Check sheet for the modelled part. Datum: model origin and axes. Units: mm. Face numbers are marked on the shaded views. A direction names the side the tool comes from. Round coordinates to 2 decimals unless told otherwise and drop trailing zeros. Loops run counter-clockwise (first coordinate to the right, second up) from the corner with the lowest first, then second, coordinate; pieces in that order, holes last. Notation, with made-up numbers: (45.25, 14) -> (99.25, 14) arc R7 ccw to (99.25, 26) -> close; hole circle Ø8 at (-3, -20). An arc over 180 degrees is marked (long way). Use one line per item in the form item = value. Start each with the question number.
(1) Material ranges on probe 1 along Y at (x, z) = (-8.5, 9.75); probe 2 along Z at (x, y) = (6, 20.5); probe 3 along Z at (x, y) = (8, 27.5), recorded low to high. Write a range as [from, to].
(2) Sectioned sample at B-B (y = 41). Record the cut outline in (x, z), and give its area (3 significant figures).
(3) Go/stop test with flat-tipped pins: pin 1 (10 mm diameter, centred on y = 20, z = 0.5, fed in from +X); pin 2 (12 mm diameter, centred on y = 39.5, z = -0.5, fed in from +X); pin 3 (2 mm diameter, centred on y = 35.5, z = -0.5, fed in from +X); pin 4 (14.5 mm diameter, centred on x = 8, z = 1, fed in from +Y). Record where each tip stops, or that it passes through.
(4) Set-up check for the marked faces 1, 2 and 3: record each of +Z, -Z, +X, -X, +Y, -Y from which the full face is reachable in a straight line by a thin tool's end or side.
(5) Sectioned sample at D-D (x = 10). Record the cut outline in (y, z).
(6) Draft check along Z on the marked faces 4, 5 and 6. Enter one of: released by +Z, released by -Z, zero draft, split by the parting line, or undercut.
(7) Sectioned sample at C-C (z = -2.25). Record the cut outline in (x, y).
(8) Sectioned sample at A-A (x = 3). Record the cut outline in (y, z).
from build123d import *

# Parameters (mm, degrees)
EXTRUDE_1_DEPTH = 3
EXTRUDE_START   = -3
EXTRUDE_2_DEPTH = 63
EXTRUDE_3_DEPTH = 3


with BuildPart() as part:
    # 草图1 → 凸台-拉伸1 (new body)
    with BuildSketch(Plane(origin=(0, 0, 0), x_dir=(1, 0, 0), z_dir=(0, 1, 0))):
        Polygon((14.549226784, 0), (7.274613392, 12.6), (-7.274613392, 12.6), (-14.549226784, 0), (-7.274613392, -12.6), (7.274613392, -12.6), align=None)
        Polygon((-8.775724092, 0), (-4.387862046, -7.6), (4.387862046, -7.6), (8.775724092, 0), (4.387862046, 7.6), (-4.387862046, 7.6), align=None, mode=Mode.SUBTRACT)
    extrude(amount=EXTRUDE_1_DEPTH)

    # 草图2 → 凸台-拉伸2 (add)
    with BuildSketch(Plane(origin=(0, 3, 0), x_dir=(1, 0, 0), z_dir=(0, 1, 0)).offset(EXTRUDE_START)):
        Polygon((-12.85862786, 6.92820323), (-16.85862786, 0), (-12.85862786, -6.92820323), (-11.126577053, -5.92820323), (-14.549226784, 0), (-11.126577053, 5.92820323), align=None)
        Polygon((8.42931393, 14.6), (0.42931393, 14.6), (0.42931393, 12.6), (7.274613392, 12.6), (10.697263123, 6.67179677), (12.42931393, 7.67179677), align=None)
        Polygon((0.42931393, -12.6), (0.42931393, -14.6), (8.42931393, -14.6), (12.42931393, -7.67179677), (10.697263123, -6.67179677), (7.274613392, -12.6), align=None)
    extrude(amount=EXTRUDE_2_DEPTH)

    # 草图2<3> → 凸台-拉伸3 (add)
    with BuildSketch(Plane(origin=(0, 3, 0), x_dir=(1, 0, 0), z_dir=(0, 1, 0))):
        Polygon((-8.42931393, 14.6), (-12.85862786, 6.92820323), (-11.126577053, 5.92820323), (-7.274613392, 12.6), (0.42931393, 12.6), (0.42931393, 14.6), align=None)
        Polygon((10.697263123, -6.67179677), (12.42931393, -7.67179677), (16.85862786, 0), (12.42931393, 7.67179677), (10.697263123, 6.67179677), (14.549226784, 0), align=None)
        Polygon((-11.126577053, -5.92820323), (-12.85862786, -6.92820323), (-8.42931393, -14.6), (0.42931393, -14.6), (0.42931393, -12.6), (-7.274613392, -12.6), align=None)
    extrude(amount=-EXTRUDE_3_DEPTH)


solid = part.part
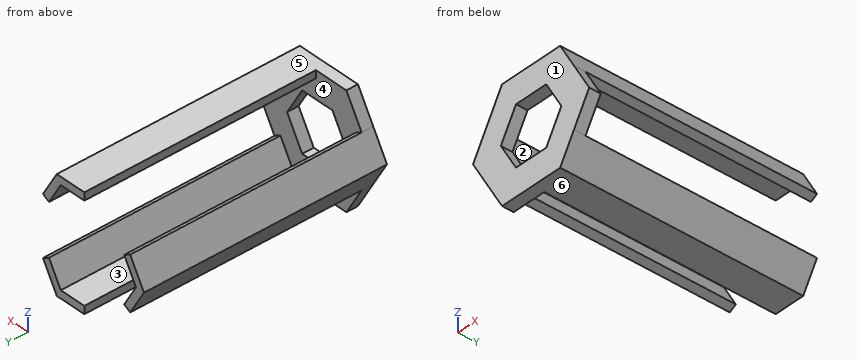
Checks:
q1.probe_1 = [0, 3]
q1.probe_2 = [-14.6, -12.6], [12.6, 14.6]
q1.probe_3 = [-14.6, -11.34], [11.34, 14.6]
q2.outline = (-16.86, 0) -> (-12.86, -6.93) -> (-11.13, -5.93) -> (-14.55, 0) -> (-11.13, 5.93) -> (-12.86, 6.93) -> close; (0.43, -14.6) -> (8.43, -14.6) -> (12.43, -7.67) -> (10.7, -6.67) -> (7.27, -12.6) -> (0.43, -12.6) -> close; (0.43, 12.6) -> (7.27, 12.6) -> (10.7, 6.67) -> (12.43, 7.67) -> (8.43, 14.6) -> (0.43, 14.6) -> close
q2.area = 89.1 mm2
q3.pin_1 = -11.37
q3.pin_2 = -11.13
q3.pin_3 = -13.68
q3.pin_4 = 63
q4.face_1 = +Z, -Z, +X, -X, -Y
q4.face_2 = +X, +Y
q4.face_3 = -X, +Y
q5.outline = (0, -11.88) -> (63, -11.88) -> (63, -7.88) -> (3, -7.88) -> (3, 7.88) -> (63, 7.88) -> (63, 11.88) -> (0, 11.88) -> close
q6.face_4 = undercut
q6.face_5 = released by +Z
q6.face_6 = released by -Z
q7.outline = (-15.56, 0) -> (-7.48, 0) -> (-7.48, 3) -> (-13.25, 3) -> (-13.25, 63) -> (-15.56, 63) -> close; (7.48, 0) -> (15.56, 0) -> (15.56, 3) -> (7.48, 3) -> close
q8.outline = (0, -14.6) -> (63, -14.6) -> (63, -12.6) -> (3, -12.6) -> (3, -7.6) -> (0, -7.6) -> close; (0, 7.6) -> (3, 7.6) -> (3, 12.6) -> (63, 12.6) -> (63, 14.6) -> (0, 14.6) -> close
